```python
from build123d import *

# Parameters (mm, degrees)
SKETCH_1_R                    = 5
SKETCH_1_R_2                  = 11
EXTRUDE_1_DEPTH               = 70
EXTRUDE_3_DEPTH               = 20
SKETCH_5_R                    = 11
SKETCH_5_R_2                  = 2
CUT_EXTRUDE_3_DEPTH           = 12
FILLET_2_R                    = 5
FILLET_1_R                    = 2
SKETCH_18_R                   = 11
CUT_EXTRUDE_8_DEPTH           = 4
SKETCH_20_R                   = 1.5
CUT_EXTRUDE_9_DEPTH           = 66
FILLET_4_R                    = 2
CHAMFER_1_SIZE                = 0.5
CHAMFER_2_SIZE                = 0.5
HOLE_START                    = 50
HOLE_WIZARD_M41_OUTLINE_R     = 2.4
HOLE_WIZARD_M41_DEPTH         = 20
HOLE_START_2                  = 65.6
HOLE_WIZARD_M41_2_OUTLINE_R   = 4
HOLE_WIZARD_M41_2_OUTLINE_R_2 = 2.4
HOLE_WIZARD_M41_2_DEPTH       = 4.4
HOLE_WIZARD_M42_D             = 4.8
HOLE_WIZARD_M42_CBORE_D       = 8
HOLE_WIZARD_M42_CBORE_DEPTH   = 4.4
CUT_EXTRUDE_11_DEPTH          = 3
CUT_EXTRUDE_12_DEPTH          = 3
CUT_EXTRUDE_14_REACH          = 147.097
SKETCH_35_W                   = 35
SKETCH_35_H                   = 60
FILLET_6_R                    = 10
FILLET_7_R                    = 15
FILLET_8_R                    = 15


# Read off the part's stored shape, not the designer's step: Цековка для  винта с внутренним шестигранником M41
with BuildPart() as part:
    # Эскиз1 → Бобышка-Вытянуть1 (new body)
    with BuildSketch(Plane(origin=(0, 0, 0), x_dir=(1, 0, 0), z_dir=(0, 1, 0))):
        Polygon((0, 0), (0, 38), (65, 38), (65, 12), (108, 12), (108, 0), align=None)
        with Locations(Location((51, 23, 0), (0, 0, 270))):
            Circle(SKETCH_1_R, mode=Mode.SUBTRACT)
        with Locations(Location((15, 23, 0), (0, 0, 270))):
            Circle(SKETCH_1_R_2, mode=Mode.SUBTRACT)
    extrude(amount=EXTRUDE_1_DEPTH)

    # Эскиз3 → Бобышка-Вытянуть3 (add)
    with BuildSketch(Plane.ZY):
        with BuildLine():
            Line((0, 70), (29, 70))
            Line((29, 70), (29, 60.5))
            Line((29, 60.5), (19.979130372, 60.5))
            ThreePointArc((19.979130372, 60.5), (8, 60), (19.979130372, 59.5))
            Line((19.979130372, 59.5), (29, 59.5))
            Line((29, 59.5), (29, 50))
            Line((29, 50), (0, 50))
            Line((0, 50), (0, 70))
        make_face()
        with BuildLine():
            Line((29, 0), (0, 0))
            Line((0, 0), (0, 20))
            Line((0, 20), (29, 20))
            Line((29, 20), (29, 10.5))
            Line((29, 10.5), (19.979130372, 10.5))
            ThreePointArc((19.979130372, 10.5), (8, 10), (19.979130372, 9.5))
            Line((19.979130372, 9.5), (29, 9.5))
            Line((29, 9.5), (29, 0))
        make_face()
    extrude(amount=-EXTRUDE_3_DEPTH)

    # Эскиз5 → Вырез-Вытянуть3 (cut)
    with BuildSketch(Plane(origin=(0, 0, -12), x_dir=(-1, 0, 0), z_dir=(0, 0, -1))):
        with Locations((-86.5, 35)):
            Circle(SKETCH_5_R)
        with Locations((-102, 19.5)):
            Circle(SKETCH_5_R_2)
        with Locations((-71, 19.5)):
            Circle(SKETCH_5_R_2)
        with Locations((-71, 50.5)):
            Circle(SKETCH_5_R_2)
        with Locations((-102, 50.5)):
            Circle(SKETCH_5_R_2)
    extrude(amount=-CUT_EXTRUDE_3_DEPTH, mode=Mode.SUBTRACT)

    # Скругление2
    fillet_2_edges = [part.edges().sort_by_distance(p)[0] for p in [
        (97.5, 35, 0),
    ]]
    fillet(fillet_2_edges, radius=FILLET_2_R)

    # Скругление1
    fillet_1_edges = [part.edges().sort_by_distance(p)[0] for p in [
        (97.5, 35, -12),
    ]]
    fillet(fillet_1_edges, radius=FILLET_1_R)

    # Эскиз18 → Вырез-Вытянуть8 (cut)
    with BuildSketch(Plane(origin=(0, 70, 0), x_dir=(1, 0, 0), z_dir=(0, 1, 0))):
        with Locations(Location((51, 23, 0), (0, 0, 270))):
            Circle(SKETCH_18_R)
    extrude(amount=-CUT_EXTRUDE_8_DEPTH, mode=Mode.SUBTRACT)

    # Эскиз20 → Вырез-Вытянуть9 (cut)
    with BuildSketch(Plane(origin=(0, 66, 0), x_dir=(1, 0, 0), z_dir=(0, 1, 0))):
        with Locations(Location((43, 23, 0), (0, 0, 270))):
            Circle(SKETCH_20_R)
        with Locations(Location((59, 23, 0), (0, 0, 270))):
            Circle(SKETCH_20_R)
        with Locations(Location((51, 31, 0), (0, 0, 270))):
            Circle(SKETCH_20_R)
        with Locations(Location((51, 15, 0), (0, 0, 270))):
            Circle(SKETCH_20_R)
    extrude(amount=-CUT_EXTRUDE_9_DEPTH, mode=Mode.SUBTRACT)

    # Скругление4
    fillet_4_edges = [part.edges().sort_by_distance(p)[0] for p in [
        (51, 70, -34),
    ]]
    fillet(fillet_4_edges, radius=FILLET_4_R)

    # Фаска1
    chamfer_1_edges = [part.edges().sort_by_distance(p)[0] for p in [
        (15, 70, -34),
    ]]
    chamfer(chamfer_1_edges, length=CHAMFER_1_SIZE)

    # Фаска2
    chamfer_2_edges = [part.edges().sort_by_distance(p)[0] for p in [
        (15, 0, -34),
    ]]
    chamfer(chamfer_2_edges, length=CHAMFER_2_SIZE)

    # Цековка для  винта с внутренним шестигранником M41 outline → Цековка для  винта с внутренним шестигранником M41 (cut)
    with BuildSketch(Plane(origin=(0, 0, 0), x_dir=(1, 0, 0), z_dir=(0, 1, 0)).offset(HOLE_START)):
        with Locations((10, -24)):
            Circle(HOLE_WIZARD_M41_OUTLINE_R)
    extrude(amount=HOLE_WIZARD_M41_DEPTH, mode=Mode.SUBTRACT)

    # Hole Wizard M41 2 outline → Hole Wizard M41 2 (cut)
    with BuildSketch(Plane(origin=(0, 0, 0), x_dir=(1, 0, 0), z_dir=(0, 1, 0)).offset(HOLE_START_2)):
        with Locations((10, -24)):
            Circle(HOLE_WIZARD_M41_2_OUTLINE_R)
        with Locations((10, -24)):
            Circle(HOLE_WIZARD_M41_2_OUTLINE_R_2, mode=Mode.SUBTRACT)
    extrude(amount=HOLE_WIZARD_M41_2_DEPTH, mode=Mode.SUBTRACT)

    # Цековка для  винта с внутренним шестигранником M42 (through all)
    with Locations(Plane(origin=(0, 0, 0), x_dir=(-1, 0, 0), z_dir=(0, -1, 0))):
        with Locations((-10, -24)):
            CounterBoreHole(HOLE_WIZARD_M42_D / 2, HOLE_WIZARD_M42_CBORE_D / 2, HOLE_WIZARD_M42_CBORE_DEPTH)

    # Эскиз29 → Вырез-Вытянуть11 (cut)
    with BuildSketch(Plane(origin=(0, 20, 0), x_dir=(1, 0, 0), z_dir=(0, 1, 0))):
        Polygon((7.979274058, -27.5), (12.020725942, -27.5), (14.041451884, -24), (12.020725942, -20.5), (7.979274058, -20.5), (5.958548116, -24), align=None)
    extrude(amount=-CUT_EXTRUDE_11_DEPTH, mode=Mode.SUBTRACT)

    # Эскиз34 → Вырез-Вытянуть12 (cut)
    with BuildSketch(Plane(origin=(0, 50, 0), x_dir=(-1, 0, 0), z_dir=(0, -1, 0))):
        Polygon((-7.979274058, -27.5), (-12.020725942, -27.5), (-14.041451884, -24), (-12.020725942, -20.5), (-7.979274058, -20.5), (-5.958548116, -24), align=None)
    extrude(amount=-CUT_EXTRUDE_12_DEPTH, mode=Mode.SUBTRACT)

    # Вырез-Вытянуть14: up to this face of the body (flat: up to its plane)
    cut_extrude_14_end = Plane(part.part.faces().sort_by_distance((100.321522976, 35, -12))[0])
    # Эскиз35 → Вырез-Вытянуть14 (cut, up to the picked face)
    with BuildSketch(Plane(origin=(0, 0, -38), x_dir=(-1, 0, 0), z_dir=(0, 0, -1)), mode=Mode.PRIVATE) as cut_extrude_14_sk1:
        with Locations((-47.5, 30)):
            Rectangle(SKETCH_35_W, SKETCH_35_H)
    cut_extrude_14_tool1 = split(extrude(cut_extrude_14_sk1.sketch, amount=-CUT_EXTRUDE_14_REACH, mode=Mode.PRIVATE), bisect_by=cut_extrude_14_end, keep=Keep.BOTH, mode=Mode.PRIVATE)
    add(cut_extrude_14_tool1.solids().sort_by(Axis((47.5, 30, -38), (0, 0, 1)))[0], mode=Mode.SUBTRACT)

    # Скругление6
    fillet_6_edges = [part.edges().sort_by_distance(p)[0] for p in [
        (65, 65, -38),
    ]]
    fillet(fillet_6_edges, radius=FILLET_6_R)

    # Скругление7
    fillet_7_edges = [part.edges().sort_by_distance(p)[0] for p in [
        (30, 30, -38),
    ]]
    fillet(fillet_7_edges, radius=FILLET_7_R)

    # Скругление8
    fillet_8_edges = [part.edges().sort_by_distance(p)[0] for p in [
        (0, 35, -38),
    ]]
    fillet(fillet_8_edges, radius=FILLET_8_R - 0.0001)  # a hair under: the kernel refuses the full size


solid = part.part
```
Check sheet for the modelled part. Datum: model origin and axes. Units: mm. A direction names the side the tool comes from. Coordinates: 2 decimals unless noted, no trailing zeros. Order: outer loops, then holes, each group sorted by start corner. A loop starts at its lowest first (then second) coordinate and runs counter-clockwise, first axis right, second up. Notation, with made-up numbers: M 1,72 L 39,72 A17 ccw 39,84 Z; hole C -38.5,13 d2. An arc over 180 degrees is marked long. Write each question's results on one line, items separated by ' | '. Start each with the question number.
1. Material ranges on probe 1 along X at (y, z) = (54, -22.5); probe 2 along X at (y, z) = (63, -23); probe 3 along Y at (x, z) = (102, -4.5), recorded low to high.
2. Go/stop test with flat-tipped pins: P1, Ø4, axis at x = 10, z = 25, coming from the +Y side; P2, Ø5.5, axis at x = 10, z = 24, coming from the -Y side; P3, Ø1, axis at x = 19.5, y = 40, coming from the -Z side. Record where each tip stops, or that it passes through.
3. Access from +Z, -Z, +X, -X, +Y, -Y to the whole of each face (thin tool, end or side, straight path). Record for faces 5 (the face through (10, 20, 14)), 6 (the face through (10, 19, 27.5)), 7 (the face through (60.275, 67.014, -17.086)).
4. Mould release check, pull along Y, two halves, no side actions. Record for faces 1 (the face through (4.51, 35.49, -33.72)), 2 (the face through (7.6, 9.5, 25.4)), 3 (the face through (8, 4.4, 26)), 4 (the face through (7, 18.5, 22.2)): +Y half, -Y half, draft (parallel to the pull), parting line (faces both ways), or undercut.
5. Cross-section at A-A on y = 35. State how many separate pieces and enclosed holes the cut face has, and give its area (3 significant figures).
6. Cross-section at D-D on x = 67.5. Record the cut outline in (y, z), and give its area (3 significant figures).
Checks:
1) probe 1: x = 0 to 4.01, 25.99 to 30 | probe 2: x = 0 to 4, 26 to 41.5, 44.5 to 46, 56 to 57.5, 60.5 to 65 | probe 3: y = 0 to 17.5, 21.5 to 48.5, 52.5 to 70
2) P1: stops at y = 65.6 | P2: stops at y = 4.4 | P3: stops at z = -37.46
3) face 5: +Z, +X, -X | face 6: none | face 7: +Y
4) face 1: draft | face 2: undercut | face 3: -Y half | face 4: undercut
5) separate pieces: 2 | enclosed holes: 1 | area: 1,320 mm²
6) outline: M 0,-12 L 70,-12 L 70,0 L 0,0 Z | area: 840 mm²
